Build history of the part. All positions in model axes, mm. A direction names the side the tool comes from. Give positions to 0.01 mm unless a question says otherwise; leave off trailing zeros. Order: outer loops, then holes, each group sorted by start corner. A loop starts at its lowest first (then second) coordinate and runs counter-clockwise, first axis right, second up. Notation, with made-up numbers: (45.5, 58) - (87.5, 58) arc R17 cw to (87.5, 89) - close; hole circle Ø8 at (73, 36.25). An arc over 180 degrees is marked (long way). One line per item, written item: value.
```python
from build123d import *

# Parameters (mm, degrees)
F1_DEPTH = 50.8
F2_R     = 13.716
F3_DEPTH = 25.4
F4_R     = 12.7
F5_DEPTH = 35.56


with BuildPart() as f1:
    # F0 (on Top) → F1 (new body)
    with BuildSketch(Plane.XY):
        Polygon((25.4, -25.4), (-25.4, 25.4), (-25.4, -25.4), align=None)
    extrude(amount=F1_DEPTH)

    # F2 (on face) → F3 (join)
    with BuildSketch(Plane(origin=(0, 0, 0), x_dir=(-0.7071067812, 0.7071067812, 0), z_dir=(0.7071067812, 0.7071067812, 0))):
        with Locations((0, 25.4)):
            Circle(F2_R)
    extrude(amount=F3_DEPTH)

    # F4 (on face) → F5 (cut)
    with BuildSketch(Plane(origin=(17.9605122421, 17.9605122421, 0), x_dir=(-0.7071067812, 0.7071067812, 0), z_dir=(0.7071067812, 0.7071067812, 0))):
        with Locations((0, 25.4)):
            Circle(F4_R)
    extrude(amount=-F5_DEPTH, mode=Mode.SUBTRACT)


solid = f1.part
```
(1) Pull direction Y, two halves, no side cores. Call faces 3 (the face through (-25.4, 0, 25)), 4 (the face through (0, -25.4, 25)), 5 (the face through (10.1, 7.6, 39)): +Y half, -Y half, draft (parallel to the pull), parting line (faces both ways), or undercut.
Completed:
face 3: draft
face 4: -Y half
face 5: undercut
(2) Drill centre lines: line 1 (Z direction, x = 8.5, y = -0.5); line 2 (Y direction, x = 12, z = 14.5); line 3 (Z direction, x = 6, y = 3). Where is each one in solid material? Low to high.
Completed:
line 1: 13.25 to 14.41, 36.39 to 37.55
line 2: -25.4 to -12, 0.23 to 2.78, 21.22 to 23.77
line 3: 11.85 to 12.88, 37.92 to 38.95
(3) Pin check, flat tips, straight feed: P1, Ø6, axis at x = 6.5, y = 8, coming from the -Z side; P2, Ø3, axis at y = 17.5, z = 30.5, coming from the +X side; P3, Ø10, axis at y = -11.5, z = 42.5, coming from the +X side. Stop position of each tip, or through.
Completed:
P1: z = 11.68
P2: x = 2.87
P3: x = 16.5
(4) Slice it at A-A, the plane z = 14. Give the cut face in (x, y), and give its area (3 significant figures).
Completed:
outline: (-25.4, -25.4) - (25.4, -25.4) - (5.39, -5.39) - (23.35, 12.57) - (21.92, 14) - (-3.23, -11.14) - (-11.14, -3.23) - (14, 21.92) - (12.57, 23.35) - (-5.39, 5.39) - (-25.4, 25.4) - close
area: 1,280 mm²
(5) Slice it at D-D, the plane z = 34.5. Give the cut face in (x, y), and give its area (3 significant figures).
Completed:
outline: (-25.4, -25.4) - (25.4, -25.4) - (7.26, -7.26) - (25.22, 10.7) - (24.22, 11.7) - (-0.92, -13.45) - (-13.45, -0.92) - (11.7, 24.22) - (10.7, 25.22) - (-7.26, 7.26) - (-25.4, 25.4) - close
area: 1,180 mm²
(6) Slice it at B-B, the plane y = -18.5. Give the cut face in (x, z).
Completed:
outline: (-25.4, 0) - (18.5, 0) - (18.5, 50.8) - (-25.4, 50.8) - close
(7) 3-axis set-ups, long thin cutter, end or side, ignore diameter. For faces 1 (the face through (12.26, 23.66, 15.3)), 2 (the face through (-7.06, -7.31, 25.58)): which of +Z, -Z, +X, -X, +Y, -Y reach the whole face in a straight line?
Completed:
face 1: +Z, -Z, +X, +Y
face 2: none
(8) Slice it at C-C, the plane z = 41. Give the cut face in (x, y), and give its area (3 significant figures).
Completed:
outline: (-25.4, -25.4) - (25.4, -25.4) - (-25.4, 25.4) - close
area: 1,290 mm²
